Autodesk Inventor part; units mm, degrees
ref_plane "YZ Plane" through (0, 0, 0) normal (1, 0, 0) x (0, 1, 0)
ref_plane "XZ Plane" through (0, 0, 0) normal (0, 1, 0) x (-1, 0, 0)
ref_plane "XY Plane" through (0, 0, 0) normal (0, 0, 1) x (1, 0, 0)
sketch "スケッチ1" plane through (0, 0, 0) normal (0, 0, 1) x (1, 0, 0)
  circle A0 centre (0, 0) radius 15
  dimension "d0" = 30
extrude "押し出し1" add sketch "スケッチ1" along normal blind 30
sketch "スケッチ2" plane through (0, 0, 30) normal (0, 0, 1) x (1, 0, 0)
  circle A0 centre (0, 0) radius 15
  dimension "d3" = 30
extrude "押し出し2" add sketch "スケッチ2" along normal blind 20
sketch "スケッチ4" plane through (0, 0, 0) normal (1, 0, 0) x (0, 1, 0)
  point P0 (0, 0)
sketch "スケッチ5" plane through (0, 0, 0) normal (0, 0, -1) x (-1, 0, 0)
  circle A0 centre (0, 0) radius 14
  dimension "d6" = 28
extrude "押し出し3" cut sketch "スケッチ5" against normal blind 48
sketch "スケッチ6" plane through (0, 0, 0) normal (0, 1, 0) x (-1, 0, 0)
  line L0 (15, 0) -> (-15, 0)
  arc A0 (15, 0) -> (-15, 0) centre (0, 0) ccw
extrude "押し出し4" cut sketch "スケッチ6" along normal blind 50 and the other way blind 25
sketch "スケッチ7" plane through (0, 0, 50) normal (0, 0, 1) x (1, 0, 0)
  point P0 (0, 0)
  point P1 (10, 0)
  point P2 (-10, 0)
  dimension "d14" = 10
  dimension "d15" = 10
hole "穴1" at (10, 0, 50) at (-10, 0, 50) direction (0, 0, -1) diameter 3.4 end through all
properties part number "20220524_吸引部分筒"
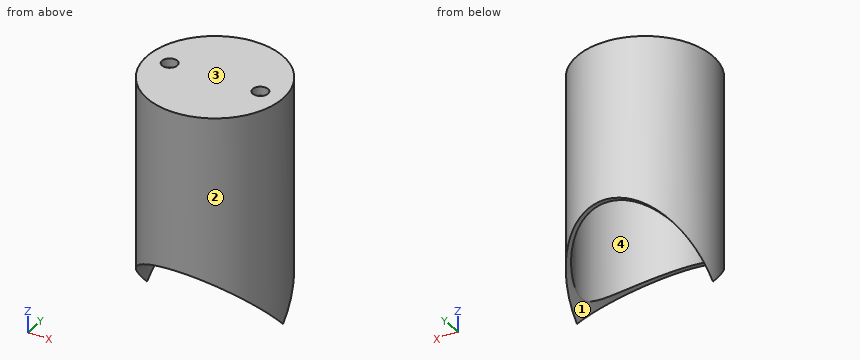
Design review of the part built by this model. Coordinates are the model's own, in mm. Face numbers are marked on the shaded views. Give positions to 0.01 mm unless a question says otherwise; leave off trailing zeros. Write each loop counter-clockwise with the first axis right and the second up, starting at its lowest first coordinate (ties: lowest second). Pieces come first, ordered by that corner, then holes. Notation, with made-up numbers: (31, 13) -> (85, 13) arc R15 cw to (85, 24) -> close; hole circle Ø2 at (51, 73.5). An arc over 180 degrees is marked (long way). Answer in a Markdown table with one row per item.
(1) Clearance check with flat-ended pins moving along their axes: pin 1 (1.5 mm diameter, centred on y = 7, z = 34, fed in from -X); pin 2 (12 mm diameter, centred on x = -4.5, y = 8, fed in from -Z); pin 3 (1.5 mm diameter, centred on y = -8, z = 5.5, fed in from -X); pin 4 (1.5 mm diameter, centred on y = -4, z = 8.5, fed in from -X). State where each tip first meets the part, or that it passes through.
Results:
| item | result |
|---|---|
| pin 1 | x = -13.64 |
| pin 2 | z = 10.89 |
| pin 3 | through |
| pin 4 | x = -14.64 |
(2) Mouldability with a two-part tool opening along X and no side actions: class the marked faces 1, 2, 3 and 4 as +X half, -X half, draft (parallel to the pull), parting line (faces both ways), or undercut.
Results:
| item | result |
|---|---|
| face 1 | undercut |
| face 2 | parting line |
| face 3 | draft |
| face 4 | undercut |
(3) To check wall thickness, follow probe 1 along X at (y, z) = (0, 48.6); probe 2 along Y at (x, z) = (0, 37); probe 3 along Z at (x, y) = (5.5, -2.75). State the ranges of each line that lie inside material, in increasing order.
Results:
| item | result |
|---|---|
| probe 1 | -15 to -11.7, -8.3 to 8.3, 11.7 to 15 |
| probe 2 | -15 to -14, 14 to 15 |
| probe 3 | 48 to 50 |
(4) Consider section B-B (x = 0). State the section outline as (y, z) points.
Results:
| item | result |
|---|---|
| outline | (-15, 15) -> (-14, 15) -> (-14, 48) -> (14, 48) -> (14, 15) -> (15, 15) -> (15, 50) -> (-15, 50) -> close |
(5) Consider section A-A (y = -1). State the section outline as (x, z) points, then the cut area to 3 significant figures.
Results:
| item | result |
|---|---|
| outline | (-14.97, 1) arc R15 cw to (-13.96, 5.48) -> (-13.96, 48) -> (-11.37, 48) -> (-11.37, 50) -> (-14.97, 50) -> close; (-8.63, 48) -> (8.63, 48) -> (8.63, 50) -> (-8.63, 50) -> close; (11.37, 48) -> (13.96, 48) -> (13.96, 5.48) arc R15 cw to (14.97, 1) -> (14.97, 50) -> (11.37, 50) -> close |
| area | 138 mm2 |
(6) Consider section D-D (z = 36). State the section outline as (x, y) points, then the cut area to 3 significant figures.
Results:
| item | result |
|---|---|
| outline | circle Ø30 at (0, 0); hole circle Ø28 at (0, 0) |
| area | 91.1 mm2 |
(7) Consider section C-C (x = -10). State the section outline as (y, z) points, then the cut area to 3 significant figures.
Results:
| item | result |
|---|---|
| outline | (-11.18, 11.18) -> (-9.8, 11.18) -> (-9.8, 48) -> (-1.7, 48) -> (-1.7, 50) -> (-11.18, 50) -> close; (1.7, 48) -> (9.8, 48) -> (9.8, 11.18) -> (11.18, 11.18) -> (11.18, 50) -> (1.7, 50) -> close |
| area | 140 mm2 |
